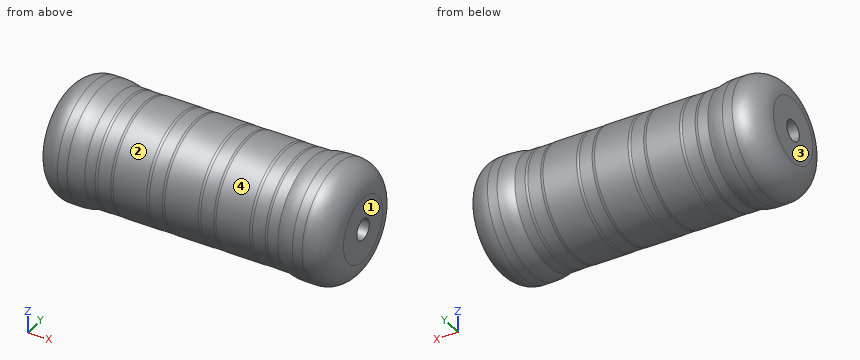
from build123d import *

# Parameters (mm, degrees)
FILLET2_R          = 1
FILLET10_R         = 0.5
FILLET11_R         = 2
SKETCH3_R          = 0.4
CUT_EXTRUDE2_DEPTH = 16


with BuildPart() as part:
    # Sketch2 → Revolve1 (revolve)
    with BuildSketch(Plane.XY, mode=Mode.PRIVATE) as revolve1_sk:
        Polygon((-6.558139535, 2.25), (-6.558139535, 0), (4.941860465, 0), (4.941860465, 2.25), (2.941860465, 2.25), (2.941860465, 2.15), (2.441860465, 2.15), (2.441860465, 2.14), (1.941860465, 2.14), (1.941860465, 2.15), (1.442088765, 2.15), (0.441860465, 2.15), (0.441860465, 2.14), (-0.058139535, 2.14), (-0.058139535, 2.15), (-1.558139535, 2.15), (-1.558139535, 2.14), (-2.058139535, 2.14), (-2.058139535, 2.15), (-3.558139535, 2.15), (-3.558139535, 2.14), (-4.058139535, 2.14), (-4.058139535, 2.15), (-4.558139535, 2.15), (-4.558139535, 2.25), align=None)
    revolve(revolve1_sk.sketch.rotate(Axis((-6.558139535, 0, 0), (1, 0, 0)), 180), axis=Axis((-6.558139535, 0, 0), (1, 0, 0)))

    # Fillet2
    fillet2_edges = [part.edges().sort_by_distance(p)[0] for p in [
        (-6.558139535, 2.25, 0),
        (4.941860465, 2.25, 0),
    ]]
    fillet(fillet2_edges, radius=FILLET2_R)

    # Fillet10
    # the kernel refuses this fillet: 0.5 mm, written as the material it takes off along each edge
    with BuildSketch(Plane(origin=(-4.058139535, 0, 0), x_dir=(0, -1, 0), z_dir=(0, 0, 1))) as fillet10_piece_1:
        with BuildLine():
            CenterArc((1.65, -0.099498744), FILLET10_R, 0, 11.478340955)
            Line((2.14, 0), (2.1498, 0.001989975))
            ThreePointArc((2.1498, 0.001989975), (2.145, 0.01), (2.15, 0.01))
            Line((2.15, 0.01), (2.16, 0))
            Line((2.16, 0), (2.16, -0.099498744))
            Line((2.16, -0.099498744), (2.15, -0.099498744))
        make_face()
    revolve(axis=Axis((-4.058139535, 0, 0), (1, 0, 0)), mode=Mode.SUBTRACT)
    with BuildSketch(Plane(origin=(-3.558139535, 0, 0), x_dir=(0, -1, 0), z_dir=(0, 0, 1))) as fillet10_piece_2:
        with BuildLine():
            CenterArc((1.65, 0.099498744), FILLET10_R, 348.521659045, 11.478340955)
            Line((2.15, 0.099498744), (2.16, 0.099498744))
            Line((2.16, 0.099498744), (2.16, 0))
            Line((2.16, 0), (2.15, -0.01))
            ThreePointArc((2.15, -0.01), (2.145, -0.01), (2.1498, -0.001989975))
            Line((2.1498, -0.001989975), (2.14, 0))
        make_face()
    revolve(axis=Axis((-3.558139535, 0, 0), (1, 0, 0)), mode=Mode.SUBTRACT)
    with BuildSketch(Plane(origin=(-2.058139535, 0, 0), x_dir=(0, -1, 0), z_dir=(0, 0, 1))) as fillet10_piece_3:
        with BuildLine():
            CenterArc((1.65, -0.099498744), FILLET10_R, 0, 11.478340955)
            Line((2.14, 0), (2.1498, 0.001989975))
            ThreePointArc((2.1498, 0.001989975), (2.145, 0.01), (2.15, 0.01))
            Line((2.15, 0.01), (2.16, 0))
            Line((2.16, 0), (2.16, -0.099498744))
            Line((2.16, -0.099498744), (2.15, -0.099498744))
        make_face()
    revolve(axis=Axis((-2.058139535, 0, 0), (1, 0, 0)), mode=Mode.SUBTRACT)
    with BuildSketch(Plane(origin=(-1.558139535, 0, 0), x_dir=(0, -1, 0), z_dir=(0, 0, 1))) as fillet10_piece_4:
        with BuildLine():
            CenterArc((1.65, 0.099498744), FILLET10_R, 348.521659045, 11.478340955)
            Line((2.15, 0.099498744), (2.16, 0.099498744))
            Line((2.16, 0.099498744), (2.16, 0))
            Line((2.16, 0), (2.15, -0.01))
            ThreePointArc((2.15, -0.01), (2.145, -0.01), (2.1498, -0.001989975))
            Line((2.1498, -0.001989975), (2.14, 0))
        make_face()
    revolve(axis=Axis((-1.558139535, 0, 0), (1, 0, 0)), mode=Mode.SUBTRACT)
    with BuildSketch(Plane(origin=(-0.058139535, 0, 0), x_dir=(0, -1, 0), z_dir=(0, 0, 1))) as fillet10_piece_5:
        with BuildLine():
            CenterArc((1.65, -0.099498744), FILLET10_R, 0, 11.478340955)
            Line((2.14, 0), (2.1498, 0.001989975))
            ThreePointArc((2.1498, 0.001989975), (2.145, 0.01), (2.15, 0.01))
            Line((2.15, 0.01), (2.16, 0))
            Line((2.16, 0), (2.16, -0.099498744))
            Line((2.16, -0.099498744), (2.15, -0.099498744))
        make_face()
    revolve(axis=Axis((-0.058139535, 0, 0), (1, 0, 0)), mode=Mode.SUBTRACT)
    with BuildSketch(Plane(origin=(0.441860465, 0, 0), x_dir=(0, -1, 0), z_dir=(0, 0, 1))) as fillet10_piece_6:
        with BuildLine():
            CenterArc((1.65, 0.099498744), FILLET10_R, 348.521659045, 11.478340955)
            Line((2.15, 0.099498744), (2.16, 0.099498744))
            Line((2.16, 0.099498744), (2.16, 0))
            Line((2.16, 0), (2.15, -0.01))
            ThreePointArc((2.15, -0.01), (2.145, -0.01), (2.1498, -0.001989975))
            Line((2.1498, -0.001989975), (2.14, 0))
        make_face()
    revolve(axis=Axis((0.441860465, 0, 0), (1, 0, 0)), mode=Mode.SUBTRACT)
    with BuildSketch(Plane(origin=(1.941860465, 0, 0), x_dir=(0, -1, 0), z_dir=(0, 0, 1))) as fillet10_piece_7:
        with BuildLine():
            CenterArc((1.65, -0.099498744), FILLET10_R, 0, 11.478340955)
            Line((2.14, 0), (2.1498, 0.001989975))
            ThreePointArc((2.1498, 0.001989975), (2.145, 0.01), (2.15, 0.01))
            Line((2.15, 0.01), (2.16, 0))
            Line((2.16, 0), (2.16, -0.099498744))
            Line((2.16, -0.099498744), (2.15, -0.099498744))
        make_face()
    revolve(axis=Axis((1.941860465, 0, 0), (1, 0, 0)), mode=Mode.SUBTRACT)
    with BuildSketch(Plane(origin=(2.441860465, 0, 0), x_dir=(0, -1, 0), z_dir=(0, 0, 1))) as fillet10_piece_8:
        with BuildLine():
            CenterArc((1.65, 0.099498744), FILLET10_R, 348.521659045, 11.478340955)
            Line((2.15, 0.099498744), (2.16, 0.099498744))
            Line((2.16, 0.099498744), (2.16, 0))
            Line((2.16, 0), (2.15, -0.01))
            ThreePointArc((2.15, -0.01), (2.145, -0.01), (2.1498, -0.001989975))
            Line((2.1498, -0.001989975), (2.14, 0))
        make_face()
    revolve(axis=Axis((2.441860465, 0, 0), (1, 0, 0)), mode=Mode.SUBTRACT)

    # Fillet11
    # the kernel refuses this fillet: 2 mm, written as the material it takes off along each edge
    with BuildSketch(Plane(origin=(-4.558139535, 0, 0), x_dir=(0, -1, 0), z_dir=(0, 0, 1))) as fillet11_piece_1:
        with BuildLine():
            CenterArc((0.25, -0.6244998), FILLET11_R, 0, 18.194872339)
            Line((2.15, 0), (2.25, 0))
            Line((2.25, 0), (2.25, -0.6244998))
        make_face()
    revolve(axis=Axis((-4.558139535, 0, 0), (1, 0, 0)), mode=Mode.SUBTRACT)
    with BuildSketch(Plane(origin=(2.941860465, 0, 0), x_dir=(0, -1, 0), z_dir=(0, 0, 1))) as fillet11_piece_2:
        with BuildLine():
            CenterArc((0.25, 0.6244998), FILLET11_R, 341.805127661, 18.194872339)
            Line((2.25, 0.6244998), (2.25, 0))
            Line((2.25, 0), (2.15, 0))
        make_face()
    revolve(axis=Axis((2.941860465, 0, 0), (1, 0, 0)), mode=Mode.SUBTRACT)

    # Sketch3 → Cut-Extrude2 (cut)
    with BuildSketch(Plane.ZY.offset(6.558139535)):
        with Locations(Location((0, 0, 0), (0, 0, 270))):
            Circle(SKETCH3_R)
    extrude(amount=-CUT_EXTRUDE2_DEPTH, mode=Mode.SUBTRACT)


solid = part.part
Work out the finished part from the listing and answer in its coordinate system (mm). Face numbers are marked on the shaded views. Give positions to 0.01 mm unless a question says otherwise; leave off trailing zeros. Order: outer loops, then holes, each group sorted by start corner. A loop starts at its lowest first (then second) coordinate and runs counter-clockwise, first axis right, second up. Notation, with made-up numbers: (15, 71) -> (39, 71) arc R30 cw to (39, 101) -> close; hole circle Ø9 at (-5, 0.25). An arc over 180 degrees is marked (long way). Answer as a JSON object with one key per item and string values. Group by question number.
1. Consider line 1 along Z through (x, y) = (2.75, 0); line 2 along Y through (x, z) = (-4.75, -0.1); line 3 along X through (y, z) = (-1.5, 0.3). Determine where each line is inside the solid, lowest interval first. Write a range as [from, to].
2. Flat-ended cylindrical pins translate along their axes: pin 1 Ø1 at (x, y) = (1.5, 0) entering from -Z; pin 2 Ø1 at (x, y) = (2, 1) entering from +Z. Find the tip coordinate at first contact, or state that the pin passes through.
3. Section A-A on x = 2.75 is taken. Determine the outline of the cut face in (y, z), plus the area to 3 significant figures.
4. The mould has two halves that part along X. Classify the marked faces 1, 2, 3 and 4: released by +X, released by -X, zero draft, split by the parting line, or undercut.
Result sheet:
{
 "1": {"line 1": "z = [-2.15, -0.4], [0.4, 2.15]", "line 2": "y = [-2.2, -0.39], [0.39, 2.2]", "line 3": "x = [-6.52, 4.9]"},
 "2": {"pin 1": "stops at z = -2.15", "pin 2": "stops at z = 2.09"},
 "3": {"outline": "circle Ø4.3 at (0, 0); hole circle Ø0.8 at (0, 0)", "area": "14.0 mm^2"},
 "4": {"face 1": "released by +X", "face 2": "undercut", "face 3": "released by -X", "face 4": "undercut"}
}
